from build123d import *

# Parameters (mm, degrees)
SKETCH4_W           = 6.4
SKETCH4_H           = 40
SKETCH4_W_2         = 5.4
SKETCH4_W_3         = 7.5
BOSS_EXTRUDE4_DEPTH = 5
SKETCH6_W           = 5.4
SKETCH6_H           = 40
SKETCH6_W_2         = 7.5
BOSS_EXTRUDE5_DEPTH = 15
SKETCH7_R           = 3.2
CUT_EXTRUDE2_DEPTH  = 73.625684162
CUT_EXTRUDE3_REACH  = 74.626
CUT_EXTRUDE4_REACH  = 90.566
CUT_EXTRUDE5_REACH  = 92.449
SKETCH10_R          = 2.1
CHAMFER1_SIZE       = 2
FILLET1_R           = 4.8
SKETCH11_R          = 2
BOSS_EXTRUDE6_DEPTH = 4
BOSS_EXTRUDE7_DEPTH = 4


with BuildPart() as part:
    # Sketch4 → Boss-Extrude4 (new body)
    with BuildSketch(Plane(origin=(0, 0, 0), x_dir=(1, 0, 0), z_dir=(0, 1, 0))):
        Polygon((0, 60), (0, 0), (66, 0), (66, 60), (56, 60), (56, 50), (62, 50), (62, 10), (56, 10), (56, 20), (49.6, 20), (42.1, 20), (35.7, 20), (30.3, 20), (30.3, 60), align=None)
        with Locations((38.9, 40)):
            Rectangle(SKETCH4_W, SKETCH4_H)
        with Locations((33, 40)):
            Rectangle(SKETCH4_W_2, SKETCH4_H)
        with Locations((45.85, 40)):
            Rectangle(SKETCH4_W_3, SKETCH4_H)
        Polygon((56, 50), (56, 60), (49.6, 60), (49.6, 20), (56, 20), align=None)
        Polygon((62, 50), (56, 50), (56, 20), (56, 10), (62, 10), align=None)
    extrude(amount=BOSS_EXTRUDE4_DEPTH)

    # Sketch6 → Boss-Extrude5 (add)
    with BuildSketch(Plane(origin=(0, 5, 0), x_dir=(1, 0, 0), z_dir=(0, 1, 0))):
        with Locations((33, 40)):
            Rectangle(SKETCH6_W, SKETCH6_H)
        with Locations((45.85, 40)):
            Rectangle(SKETCH6_W_2, SKETCH6_H)
        Polygon((62, 50), (56, 50), (56, 20), (56, 10), (62, 10), align=None)
    boss_extrude5 = extrude(amount=BOSS_EXTRUDE5_DEPTH)

    # Sketch7 → Cut-Extrude2 (cut, through all)
    with BuildSketch(Plane.ZY.offset(-30.3)):
        with Locations(Location((-40, 12.8, 0), (0, 0, 180))):
            Circle(SKETCH7_R)
    cut_extrude2 = extrude(amount=-CUT_EXTRUDE2_DEPTH, mode=Mode.SUBTRACT)

    # Cut-Extrude3: up to this face of the body (flat: up to its plane)
    cut_extrude3_end = Plane(part.part.faces().sort_by_distance((49.6, 12.5, -20.427200187))[0])
    # Sketch8 → Cut-Extrude3 (cut, up to the picked face)
    with BuildSketch(Plane.ZY.offset(-30.3), mode=Mode.PRIVATE) as cut_extrude3_sk1:
        with BuildLine():
            Line((-60, 20), (-60, 5))
            Line((-60, 5), (-44.714360106, 18.241948989))
            ThreePointArc((-44.714360106, 18.241948989), (-42.515747134, 19.546185319), (-40, 20))
            Line((-40, 20), (-60, 20))
        make_face()
    cut_extrude3_tool1 = split(extrude(cut_extrude3_sk1.sketch, amount=-CUT_EXTRUDE3_REACH, mode=Mode.PRIVATE), bisect_by=cut_extrude3_end, keep=Keep.BOTH, mode=Mode.PRIVATE)
    # Sketch8 → Cut-Extrude3 (cut, up to the picked face)
    with BuildSketch(Plane.ZY.offset(-30.3), mode=Mode.PRIVATE) as cut_extrude3_sk2:
        with BuildLine():
            Line((-35.285639894, 18.241948989), (-20, 5))
            Line((-20, 5), (-20, 20))
            Line((-20, 20), (-40, 20))
            ThreePointArc((-40, 20), (-37.484252866, 19.546185319), (-35.285639894, 18.241948989))
        make_face()
    cut_extrude3_tool2 = split(extrude(cut_extrude3_sk2.sketch, amount=-CUT_EXTRUDE3_REACH, mode=Mode.PRIVATE), bisect_by=cut_extrude3_end, keep=Keep.BOTH, mode=Mode.PRIVATE)
    cut_extrude3_1 = cut_extrude3_tool1.solids().sort_by(Axis((30.3, 15.029403, -54.154339), (1, 0, 0)))[0]
    add(cut_extrude3_1, mode=Mode.SUBTRACT)
    cut_extrude3_2 = cut_extrude3_tool2.solids().sort_by(Axis((30.3, 15.029403, -25.845661), (1, 0, 0)))[0]
    add(cut_extrude3_2, mode=Mode.SUBTRACT)
    cut_extrude3 = cut_extrude3_1 + cut_extrude3_2  # Cut-Extrude3 as one shape, for the pattern or mirror that repeats it

    # Sketch9 → Cut-Extrude4 (cut, up to next)
    with BuildSketch(Plane(origin=(62, 0, 0), x_dir=(0, 0, -1), z_dir=(1, 0, 0)), mode=Mode.PRIVATE) as cut_extrude4_sk1:
        with BuildLine():
            ThreePointArc((36.619205024, 19.156903753), (38.257832819, 19.786047059), (40, 20))
            Line((40, 20), (10, 20))
            Line((10, 20), (10, 5))
            Line((10, 5), (36.619205024, 19.156903753))
        make_face()
    cut_extrude4_tool1 = extrude(cut_extrude4_sk1.sketch, amount=-CUT_EXTRUDE4_REACH, mode=Mode.PRIVATE) & part.part
    # Sketch9 → Cut-Extrude4 (cut, up to next)
    with BuildSketch(Plane(origin=(62, 0, 0), x_dir=(0, 0, -1), z_dir=(1, 0, 0)), mode=Mode.PRIVATE) as cut_extrude4_sk2:
        with BuildLine():
            ThreePointArc((40, 20), (44.259746459, 18.604701552), (46.868488023, 14.959600029))
            Line((46.868488023, 14.959600029), (50, 5))
            Line((50, 5), (50, 20))
            Line((50, 20), (40, 20))
        make_face()
    cut_extrude4_tool2 = extrude(cut_extrude4_sk2.sketch, amount=-CUT_EXTRUDE4_REACH, mode=Mode.PRIVATE) & part.part
    cut_extrude4_1 = cut_extrude4_tool1.solids().sort_by_distance((62, 15.005893, -19.424487))[0]
    add(cut_extrude4_1, mode=Mode.SUBTRACT)
    cut_extrude4_2 = cut_extrude4_tool2.solids().sort_by_distance((62, 15.504148, -47.92116))[0]
    add(cut_extrude4_2, mode=Mode.SUBTRACT)
    cut_extrude4 = cut_extrude4_1 + cut_extrude4_2  # Cut-Extrude4 as one shape, for the pattern or mirror that repeats it

    # Mirror1: Boss-Extrude5, Cut-Extrude2, Cut-Extrude3, Cut-Extrude4 across plane
    add(boss_extrude5.mirror(Plane.ZY.offset(-33)))
    add(cut_extrude2.mirror(Plane.ZY.offset(-33)), mode=Mode.SUBTRACT)
    add(cut_extrude3.mirror(Plane.ZY.offset(-33)), mode=Mode.SUBTRACT)
    add(cut_extrude4.mirror(Plane.ZY.offset(-33)), mode=Mode.SUBTRACT)

    # Sketch10 → Cut-Extrude5 (cut, up to next)
    with BuildSketch(Plane(origin=(0, 5, 0), x_dir=(1, 0, 0), z_dir=(0, 1, 0)), mode=Mode.PRIVATE) as cut_extrude5_sk1:
        with Locations(Location((5.1, 54.9, 0), (0, 0, 270))):
            Circle(SKETCH10_R)
    cut_extrude5_tool1 = extrude(cut_extrude5_sk1.sketch, amount=-CUT_EXTRUDE5_REACH, mode=Mode.PRIVATE) & part.part
    # Sketch10 → Cut-Extrude5 (cut, up to next)
    with BuildSketch(Plane(origin=(0, 5, 0), x_dir=(1, 0, 0), z_dir=(0, 1, 0)), mode=Mode.PRIVATE) as cut_extrude5_sk2:
        with Locations(Location((60.9, 54.9, 0), (0, 0, 270))):
            Circle(SKETCH10_R)
    cut_extrude5_tool2 = extrude(cut_extrude5_sk2.sketch, amount=-CUT_EXTRUDE5_REACH, mode=Mode.PRIVATE) & part.part
    # Sketch10 → Cut-Extrude5 (cut, up to next)
    with BuildSketch(Plane(origin=(0, 5, 0), x_dir=(1, 0, 0), z_dir=(0, 1, 0)), mode=Mode.PRIVATE) as cut_extrude5_sk3:
        with Locations(Location((60.9, 5.1, 0), (0, 0, 270))):
            Circle(SKETCH10_R)
    cut_extrude5_tool3 = extrude(cut_extrude5_sk3.sketch, amount=-CUT_EXTRUDE5_REACH, mode=Mode.PRIVATE) & part.part
    # Sketch10 → Cut-Extrude5 (cut, up to next)
    with BuildSketch(Plane(origin=(0, 5, 0), x_dir=(1, 0, 0), z_dir=(0, 1, 0)), mode=Mode.PRIVATE) as cut_extrude5_sk4:
        with Locations(Location((5.1, 5.1, 0), (0, 0, 270))):
            Circle(SKETCH10_R)
    cut_extrude5_tool4 = extrude(cut_extrude5_sk4.sketch, amount=-CUT_EXTRUDE5_REACH, mode=Mode.PRIVATE) & part.part
    add(cut_extrude5_tool1.solids().sort_by_distance((5.1, 5, -54.9))[0], mode=Mode.SUBTRACT)
    add(cut_extrude5_tool2.solids().sort_by_distance((60.9, 5, -54.9))[0], mode=Mode.SUBTRACT)
    add(cut_extrude5_tool3.solids().sort_by_distance((60.9, 5, -5.1))[0], mode=Mode.SUBTRACT)
    add(cut_extrude5_tool4.solids().sort_by_distance((5.1, 5, -5.1))[0], mode=Mode.SUBTRACT)

    # Chamfer1
    chamfer1_edges = [part.edges().sort_by_distance(p)[0] for p in [
        (5.1, 5, -7.2),
        (60.9, 5, -7.2),
        (60.9, 5, -57),
        (5.1, 5, -57),
    ]]
    chamfer(chamfer1_edges, length=CHAMFER1_SIZE)

    # Fillet1
    fillet1_edges = [part.edges().sort_by_distance(p)[0] for p in [
        (66, 2.5, 0),
        (0, 2.5, 0),
        (0, 2.5, -60),
        (66, 2.5, -60),
    ]]
    fillet(fillet1_edges, radius=FILLET1_R)

    # Sketch11 → Boss-Extrude6 (add)
    with BuildSketch(Plane(origin=(0, 5, 0), x_dir=(1, 0, 0), z_dir=(0, 1, 0))):
        with Locations(Location((19, 11, 0), (0, 0, 270))):
            Circle(SKETCH11_R)
        with Locations(Location((47, 11, 0), (0, 0, 270))):
            Circle(SKETCH11_R)
    extrude(amount=BOSS_EXTRUDE6_DEPTH)

    # Sketch12 → Boss-Extrude7 (add)
    with BuildSketch(Plane.ZY.offset(-4)):
        Polygon((-45.25, 9.768911087), (-45.25, 15.831088913), (-46.25, 15.831088913), (-46.25, 5), (-33.75, 5), (-33.75, 15.831088913), (-34.75, 15.831088913), (-34.75, 9.768911087), (-40, 6.737822174), align=None)
    extrude(amount=BOSS_EXTRUDE7_DEPTH)


solid = part.part
Verification items for the finished model (mm, model axes). A direction names the side the tool comes from. Round coordinates to 2 decimals unless told otherwise and drop trailing zeros. Write each loop counter-clockwise with the first axis right and the second up, starting at its lowest first coordinate (ties: lowest second). Pieces come first, ordered by that corner, then holes.
(1) Section check C-C (y = 12.8). Give the number of separate pieces and of enclosed holes in the cut face, plus the area to 3 significant figures.
Returned:
separate pieces: 10
enclosed holes: 0
area: 524 mm2
(2) Material ranges on line 1 (X direction, y = 5.25, z = -30); line 2 (Y direction, x = 18, z = -40); line 3 (X direction, y = 11.5, z = -23), recorded low to high.
Returned:
line 1: x = 4 to 10, 16.4 to 23.9, 30.3 to 35.7, 42.1 to 49.6, 56 to 62
line 2: y = 0 to 9.6, 16 to 20
line 3: x = 4 to 10, 56 to 62
(3) Mould release check, pull along Y, two halves, no side actions. Record for faces 6 (the flat face through (45.798, 11.714, -27.75)), 7 (the cylindrical face through (58.96, 10.64, -37.64)), 8 (the flat face through (42.1, 9, -40)): pulls with the +Y half, pulls with the -Y half, needs draft (parallel to the pull), parting line crosses it, or undercut.
Returned:
face 6: pulls with the +Y half
face 7: undercut
face 8: needs draft
(4) Section check A-A (x = 19). Enter the section's corners in (y, z), plus the area to 3 significant figures.
Returned:
outline: (0, -60) - (5, -60) - (18.24, -44.71) arc R7.2 ccw to (18.24, -35.29) - (5, -20) - (5, -13) - (9, -13) - (9, -9) - (5, -9) - (5, 0) - (0, 0) - close; hole circle Ø6.4 at (12.8, -40)
area: 622 mm2
(5) Section check B-B (z = -25.5). Enter the section's corners in (x, y).
Returned:
outline: (0, 0) - (66, 0) - (66, 5) - (62, 5) - (62, 13.24) - (56, 13.24) - (56, 5) - (49.6, 5) - (49.6, 9.76) - (42.1, 9.76) - (42.1, 5) - (35.7, 5) - (35.7, 9.76) - (30.3, 9.76) - (30.3, 5) - (23.9, 5) - (23.9, 9.76) - (16.4, 9.76) - (16.4, 5) - (10, 5) - (10, 13.24) - (4, 13.24) - (4, 5) - (0, 5) - close
(6) Depth check by flat-ended pin: pin 1 Ø0.5 at (x, z) = (2, -45.5) entering from +Y; pin 2 Ø8 at (x, y) = (27, 17) entering from -Z; pin 3 Ø12 at (y, z) = (16.5, -53) entering from -X. Enter the tip coordinate at first touch or a pass-through.
Returned:
pin 1: stops at y = 15.83
pin 2: stops at z = -49.07
pin 3: stops at x = 16.4
(7) Section check D-D (x = 55). Enter the section's corners in (y, z).
Returned:
outline: (0, -60) - (5, -60) - (5, 0) - (0, 0) - close
(8) Access from +Z, -Z, +X, -X, +Y, -Y to the whole of each face (thin tool, end or side, straight path). Record for faces 1 (the flat face through (49.6, 9, -40)), 2 (the flat face through (33.038, 11.714, -27.75)), 3 (the flat face through (2, 13, -34.75)), 4 (the cylindrical face through (21, 7, -11)), 5 (the flat face through (2, 10, -33.75)).
Returned:
face 1: +Z, -Z, +Y
face 2: +Z, +Y
face 3: -X, +Y
face 4: +Y
face 5: +Z, -X, +Y
